The listing builds one solid part. Answer for the finished solid, in the listing's coordinates (mm). A direction names the side the tool comes from. Coordinates: 2 decimals unless noted, no trailing zeros. Order: outer loops, then holes, each group sorted by start corner. A loop starts at its lowest first (then second) coordinate and runs counter-clockwise, first axis right, second up. Notation, with made-up numbers: (51.25, 30) - (74.25, 30) arc R19 cw to (74.25, 47) - close; hole circle Ø9 at (47.25, 34). An arc over 180 degrees is marked (long way). Use one line per item in the form item = value. Start each with the question number.
Item 1: Section D-D, the plane x = 0.75 is taken. Write down the section's boundary in (y, z), and give its area (3 significant figures).
Item 2: A tool of negligible diameter and unlimited length cuts with its end or side. For faces 1 (the flat face through (-11.112, 0, -4)), 2 (the flat face through (0, -6.049, -16)), 3 (the flat face through (0, 6.049, -16)), 4 (the flat face through (6, 0, -3.175)), from which of +Z, -Z, +X, -X, +Y, -Y can it reach the whole face along a straight path? Write none if from no direction.
Item 3: Consider line 1 along Z through (x, y) = (6.25, 8) (3 decimals); line 2 along Z through (x, y) = (8.25, -5) (3 decimals); line 3 along Y through (x, z) = (-5.5, -4). Determine where each line is inside the solid, lowest interval first. Write a range as [from, to].
Item 4: The mould has two halves that part along X. Classify faces 5 (the cylindrical face through (0, 0, -3)), 6 (the flat face through (6, 0, 3.683)), 7 (the flat face through (1.587, 0, 0)): released by +X, released by -X, zero draft, split by the parting line, or undercut.
Item 5: Section A-A, the plane x = 7.75 is taken. Write down the section's boundary in (y, z) (3 decimals), and give its area (3 significant figures).
Item 6: Section B-B, the plane y = 0 is taken. Write down the section's boundary in (x, z) (1 decimal).
Item 7: Each of these flat-tipped pins is pushed along its axis until it touches: pin 1 Ø2 at (x, z) = (-3.5, -17) entering from +Y; pin 2 Ø2 at (x, y) = (-4, -10.5) entering from -Z; pin 3 Ø2 at (y, z) = (-0.5, 0) entering from +X; pin 4 Ø7.5 at (x, y) = (-4.76, 0) entering from +Z. Where does it stop, or does it pass through?
Item 8: Section C-C, the plane z = -6 is taken. Write down the section's boundary in (x, y) (1 decimal).
from build123d import *

# Parameters (mm, degrees)
F0_W     = 22.225
F0_H     = 25.4
F1_DEPTH = 12.7
F2_W     = 9.525
F2_H     = 6.858
F6_DEPTH = 25.401
F7_W     = 12.098386
F7_H     = 6.654872
F3_DEPTH = 22.225
F4_DEPTH = 32.055872


with BuildPart() as f1:
    # F0 (on Front) → F1 (new body, symmetric)
    with BuildSketch(Plane.XZ):
        Rectangle(F0_W, F0_H)
    extrude(amount=F1_DEPTH, both=True)

    # F2 (on face) → F6 (cut, through all)
    with BuildSketch(Plane.XZ.offset(12.7)):
        with Locations((6.35, 0.254)):
            Rectangle(F2_W, F2_H)
    extrude(amount=-F6_DEPTH, mode=Mode.SUBTRACT)

    # F7 (on face) → F3 (join, through all)
    with BuildSketch(Plane.YZ.offset(11.1125)):
        with Locations((0, -16.027436)):
            Rectangle(F7_W, F7_H)
    extrude(amount=-F3_DEPTH)

    # F8 (on face) → F4 (cut, through all)
    with BuildSketch(Plane.XY.offset(12.7)):
        with BuildLine():
            Line((-9.525, 0), (0, 0))
            ThreePointArc((0, 0), (-4.7625, 4.7625), (-9.525, 0))
        make_face()
        with BuildLine():
            ThreePointArc((-9.525, 0), (-4.7625, -4.7625), (0, 0))
            Line((0, 0), (-9.525, 0))
        make_face()
    extrude(amount=-F4_DEPTH, mode=Mode.SUBTRACT)


solid = f1.part
Response:
q1.outline = (-12.7, -12.7) - (-6.05, -12.7) - (-6.05, -19.35) - (6.05, -19.35) - (6.05, -12.7) - (12.7, -12.7) - (12.7, 12.7) - (-12.7, 12.7) - close
q1.area = 726 mm2
q2.face_1 = +Z, -Z, -X, +Y, -Y
q2.face_2 = -Z, +X, -X, -Y
q2.face_3 = -Z, +X, -X, +Y
q2.face_4 = +X, +Y, -Y
q3.line_1 = [-12.7, -3.175], [3.683, 12.7]
q3.line_2 = [-19.355, -3.175], [3.683, 12.7]
q3.line_3 = [-12.7, -4.71], [4.71, 12.7]
q4.face_5 = undercut
q4.face_6 = zero draft
q4.face_7 = released by +X
q5.outline = (-12.7, -12.7) - (-6.049, -12.7) - (-6.049, -19.355) - (6.049, -19.355) - (6.049, -12.7) - (12.7, -12.7) - (12.7, -3.175) - (-12.7, -3.175) - close; (-12.7, 3.683) - (12.7, 3.683) - (12.7, 12.7) - (-12.7, 12.7) - close
q5.area = 551 mm2
q6.outline = (-11.1, -19.4) - (-9.5, -19.4) - (-9.5, 12.7) - (-11.1, 12.7) - close; (0, -19.4) - (11.1, -19.4) - (11.1, -3.2) - (1.6, -3.2) - (1.6, 3.7) - (11.1, 3.7) - (11.1, 12.7) - (0, 12.7) - close
q7.pin_1 = 6.05
q7.pin_2 = -12.7
q7.pin_3 = 1.59
q7.pin_4 = through
q8.outline = (-11.1, -12.7) - (11.1, -12.7) - (11.1, 12.7) - (-11.1, 12.7) - close; hole circle Ø9.5 at (-4.8, 0)
